Input: part model. Units: mm. Frame: model coordinates. Face numbers are marked on the shaded views. A direction names the side the tool comes from. Coordinates: 2 decimals unless noted, no trailing zeros. Loops run counter-clockwise (first coordinate to the right, second up) from the corner with the lowest first, then second, coordinate; pieces in that order, holes last. Notation, with made-up numbers: (-4.75, 25) -> (27.25, 25) arc R17 cw to (27.25, 42) -> close; hole circle Ø2 at (28, 40.5). An arc over 180 degrees is marked (long way). Answer as a JSON object with one key per item and string values.
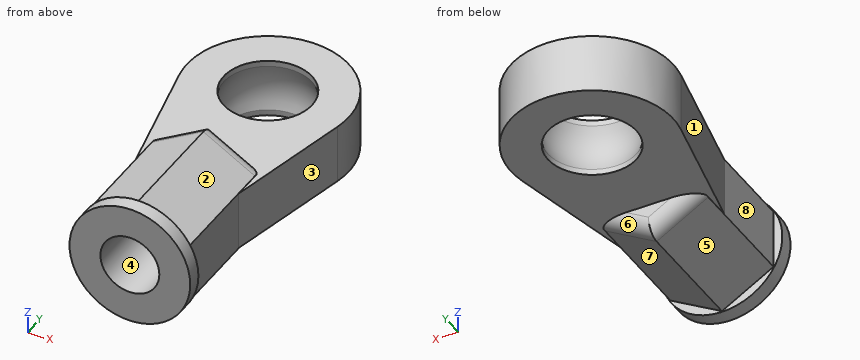
from build123d import *

# Parameters (mm, degrees)
SKETCH_R     = 3
PAD_DEPTH    = 2
PAD001_DEPTH = 9
SKETCH002_R  = 4.1
PAD002_DEPTH = 1
SKETCH003_R  = 2
POCKET_DEPTH = 6
FILLET_R     = 1


with BuildPart() as revolution:
    # Sketch004 → Revolution (revolve)
    with BuildSketch(Plane.XZ):
        with BuildLine():
            ThreePointArc((0, -3.4), (3.4, 0), (0, 3.4))
            Line((0, 3.4), (0, -3.4))
        make_face()
    revolve(axis=Axis((0, 0, 0), (0, 0, 1)))


with BuildPart() as cut:
    # Sketch → Pad (new body, symmetric)
    with BuildSketch(Plane.XY):
        with BuildLine():
            ThreePointArc((5.377475, -1.154453), (0, 5.5), (-5.377475, -1.154453))
            Line((-3.5, -9.9), (-5.377475, -1.154453))
            Line((-3.5, -15.9), (-3.5, -9.9))
            Line((3.5, -15.9), (-3.5, -15.9))
            Line((3.5, -9.9), (3.5, -15.9))
            Line((5.377475, -1.154453), (3.5, -9.9))
        make_face()
        Circle(SKETCH_R, mode=Mode.SUBTRACT)
    extrude(amount=PAD_DEPTH, both=True)

    # Sketch001 → Pad001 (new body)
    with BuildSketch(Plane.XZ.offset(15.9)):
        Polygon((3.5, 2.020726), (0, 4.041452), (-3.5, 2.020726), (-3.5, -2.020726), (0, -4.041452), (3.5, -2.020726), align=None)
    extrude(amount=-PAD001_DEPTH)

    # Sketch002 → Pad002 (new body)
    with BuildSketch(Plane.XZ.offset(15.9)):
        Circle(SKETCH002_R)
    extrude(amount=PAD002_DEPTH)

    # Sketch003 → Pocket (cut)
    with BuildSketch(Plane.XZ.offset(16.9)):
        Circle(SKETCH003_R)
    extrude(amount=-POCKET_DEPTH, mode=Mode.SUBTRACT)

    # Fillet
    fillet_edges = [cut.edges().sort_by_distance(p)[0] for p in [
        (-1.75, -6.9, 3.031089),
        (1.75, -6.9, 3.031089),
        (-1.75, -6.9, -3.031089),
        (1.75, -6.9, -3.031089),
    ]]
    fillet(fillet_edges, radius=FILLET_R)

    # Cut: cut Revolution
    add(revolution.part, mode=Mode.SUBTRACT)


solid = cut.part
1. Pin query (flat end, axial travel): P1, Ø1.2, axis at x = 1, z = 0.5, coming from the -Y side; P2, Ø5.5, axis at x = -2, y = -5.5, coming from the +Z side; P3, Ø1.5, axis at x = -3.5, z = 0.5, coming from the +Y side; P4, Ø1.5, axis at x = -4, z = 3, coming from the -Y side. Return the tip coordinate at first contact, or that it passes through.
Reply:
{"P1": "stops at y = -10.9", "P2": "stops at z = 3.88", "P3": "stops at y = 4.76", "P4": "passes through"}
2. Access query for the marked faces 1, 2, 3, 4 and 5. Directions: +Z, -Z, +X, -X, +Y, -Y. A direction counts if a zero-diameter tool reaches every point of the face in a straight line with its end or side. Return the directions, or none.
Reply:
{"face 1": "+Z, -Z, -X", "face 2": "+Z, +X, +Y", "face 3": "+Z, -Z, +X", "face 4": "-Y", "face 5": "-Z, -X, +Y"}
3. Section query D-D (x = 4.5). Return loops of the section in (y, z).
Reply:
{"outline": "(-5.24, -2) -> (3.16, -2) -> (3.16, 2) -> (-5.24, 2) -> close"}
4. Section query A-A (z = 0). Return loops of the section in (x, y).
Reply:
{"outline": "(-5.38, -1.15) -> (-3.5, -9.9) -> (-3.5, -15.9) -> (-4.1, -15.9) -> (-4.1, -16.9) -> (-2, -16.9) -> (-2, -10.9) -> (2, -10.9) -> (2, -16.9) -> (4.1, -16.9) -> (4.1, -15.9) -> (3.5, -15.9) -> (3.5, -9.9) -> (5.38, -1.15) arc R5.5 ccw (long way) to start; hole circle Ø6.8 at (0, 0)"}
5. Line query: line 1 along X through (y, z) = (0, -1.9); line 2 along Y through (x, z) = (0, 1.95); line 3 along Z through (x, y) = (-1.25, -5.5). Output: solid intervals per line, ascending.
Reply:
{"line 1": "x = -5.5 to -3, 3 to 5.5", "line 2": "y = -10.9 to -3, 3 to 5.5", "line 3": "z = -2 to 2"}
6. Section query C-C (y = -14). Return loops of the section in (x, z), plus the area to 3 significant figures.
Reply:
{"outline": "(-3.5, -2.02) -> (0, -4.04) -> (3.5, -2.02) -> (3.5, 2.02) -> (0, 4.04) -> (-3.5, 2.02) -> close; hole circle Ø4 at (0, 0)", "area": "29.9 mm2"}
7. Section query B-B (y = 0). Return loops of the section in (x, z), plus the area to 3 significant figures.
Reply:
{"outline": "(-5.5, -2) -> (-3, -2) -> (-3, -1.6) arc R3.4 cw to (-3, 1.6) -> (-3, 2) -> (-5.5, 2) -> close; (3, -2) -> (5.5, -2) -> (5.5, 2) -> (3, 2) -> (3, 1.6) arc R3.4 cw to (3, -1.6) -> close", "area": "18.3 mm2"}
8. Mould query, pull axis Y, two halves, no side actions, for the marked faces 6, 7 and 8. Classes: pulls with the +Y half, pulls with the -Y half, needs draft (parallel to the pull), parting line crosses it, or undercut.
Reply:
{"face 6": "pulls with the +Y half", "face 7": "needs draft", "face 8": "undercut"}
